The listing builds one solid part. Answer for the finished solid, in the listing's coordinates (mm). A direction names the side the tool comes from. Round coordinates to 2 decimals unless told otherwise and drop trailing zeros. Write each loop counter-clockwise with the first axis right and the second up, starting at its lowest first coordinate (ties: lowest second). Pieces come first, ordered by that corner, then holes.
Item 1: A tool of negligible diameter and unlimited length cuts with its end or side. For faces 1 (the face through (-4, -2, 0)), 2 (the face through (-6.094, -0.268, 11.944)), from which of +Z, -Z, +X, -X, +Y, -Y can it reach the whole face along a straight path? Write none if from no direction.
Item 2: Find section C-C on z = 11.25. Give the vertices of the cut face in (x, y), then the cut area to 3 significant figures.
Item 3: Find section A-A on x = 0. Give the vertices of the cut face in (y, z), then the cut area to 3 significant figures.
Item 4: Find the intervals of material crossed by probe 1 along Y at (x, z) = (0, 6.5); probe 2 along Z at (x, y) = (-3, -6); probe 3 along Y at (x, z) = (0, 12), in increasing order.
Item 5: Each of these flat-tipped pins is pushed along its axis until it touches: pin 1 (1 mm diameter, centred on y = 4, z = 5.5, fed in from -X); pin 2 (1.5 mm diameter, centred on y = 3.5, z = 4, fed in from +X); pin 3 (4 mm diameter, centred on y = 4.5, z = 7.5, fed in from +X). Where does it stop, or does it pass through?
Item 6: For a pull along Z with two mould halves and no side action, classify faces 3 (the face through (-2, -6, 16)), 4 (the face through (-1.73, 7.81, 16.99)), 5 (the face through (-4, -2, 18)) as +Z half, -Z half, draft (parallel to the pull), parting line (faces both ways), or undercut.
Item 7: Find section D-D on y = 4.5. Give the vertices of the cut face in (x, z).
Item 8: Find section B-B on y = -1.5. Give the vertices of the cut face in (x, z), then the cut area to 3 significant figures.
Autodesk Inventor part; units mm, degrees
ref_plane "YZ Plane" through (0, 0, 0) normal (1, 0, 0) x (0, 1, 0)
ref_plane "XZ Plane" through (0, 0, 0) normal (0, 1, 0) x (-1, 0, 0)
ref_plane "XY Plane" through (0, 0, 0) normal (0, 0, 1) x (1, 0, 0)
sketch "Sketch1" plane through (0, 0, 0) normal (0, 0, 1) x (1, 0, 0)
  circle A0 centre (0, 0) radius 4
  circle A1 centre (0, 0) radius 8
  circle A2 centre (0, 0) radius 6.1
  dimension "d0" = 8
  dimension "d1" = 16
  dimension "d2" = 12.2
extrude "Extrusion1" add sketch "Sketch1" along normal blind 8 contours A1 | A2
extrude "Extrusion2" add sketch "Sketch1" along normal blind 16 contours A2
sketch "Sketch2" plane through (0, 0, 16) normal (0, 0, 1) x (1, 0, 0)
  circle A0 centre (0, 0) radius 8
  circle A1 centre (0, 0) radius 4
extrude "Extrusion3" add sketch "Sketch2" along normal blind 2
properties part number "Polea" material "Aluminio 6061"
Check values:
1. face 1: -Z, +X, -X, +Y, -Y
1. face 2: none
2. outline: circle Ø12.2 at (0, 0); hole circle Ø8 at (0, 0)
2. area: 66.6 mm2
3. outline: (-8, 0) - (-4, 0) - (-4, 18) - (-8, 18) - (-8, 16) - (-6.1, 16) - (-6.1, 8) - (-8, 8) - close; (4, 0) - (8, 0) - (8, 8) - (6.1, 8) - (6.1, 16) - (8, 16) - (8, 18) - (4, 18) - close
3. area: 114 mm2
4. probe 1: y = -8 to -4, 4 to 8
4. probe 2: z = 0 to 8, 16 to 18
4. probe 3: y = -6.1 to -4, 4 to 6.1
5. pin 1: stops at x = -7.19
5. pin 2: stops at x = 7.51
5. pin 3: stops at x = 7.6
6. face 3: undercut
6. face 4: draft
6. face 5: +Z half
7. outline: (-6.61, 0) - (6.61, 0) - (6.61, 8) - (4.12, 8) - (4.12, 16) - (6.61, 16) - (6.61, 18) - (-6.61, 18) - (-6.61, 16) - (-4.12, 16) - (-4.12, 8) - (-6.61, 8) - close
8. outline: (-7.86, 0) - (-3.71, 0) - (-3.71, 18) - (-7.86, 18) - (-7.86, 16) - (-5.91, 16) - (-5.91, 8) - (-7.86, 8) - close; (3.71, 0) - (7.86, 0) - (7.86, 8) - (5.91, 8) - (5.91, 16) - (7.86, 16) - (7.86, 18) - (3.71, 18) - close
8. area: 118 mm2
